Check sheet for the drawn part. Datum: minimum x, y, z corner. Units: mm. Round coordinates to 2 decimals unless told otherwise and drop trailing zeros. Write each loop counter-clockwise with the first axis right and the second up, starting at its lowest first coordinate (ties: lowest second). Pieces come first, ordered by that corner, then holes. Notation, with made-up numbers: (79, 18) -> (138, 18) arc R13 cw to (138, 28) -> close; hole circle Ø10 at (-3.5, 0.5). An arc over 180 degrees is marked (long way). One line per item, written item: value.
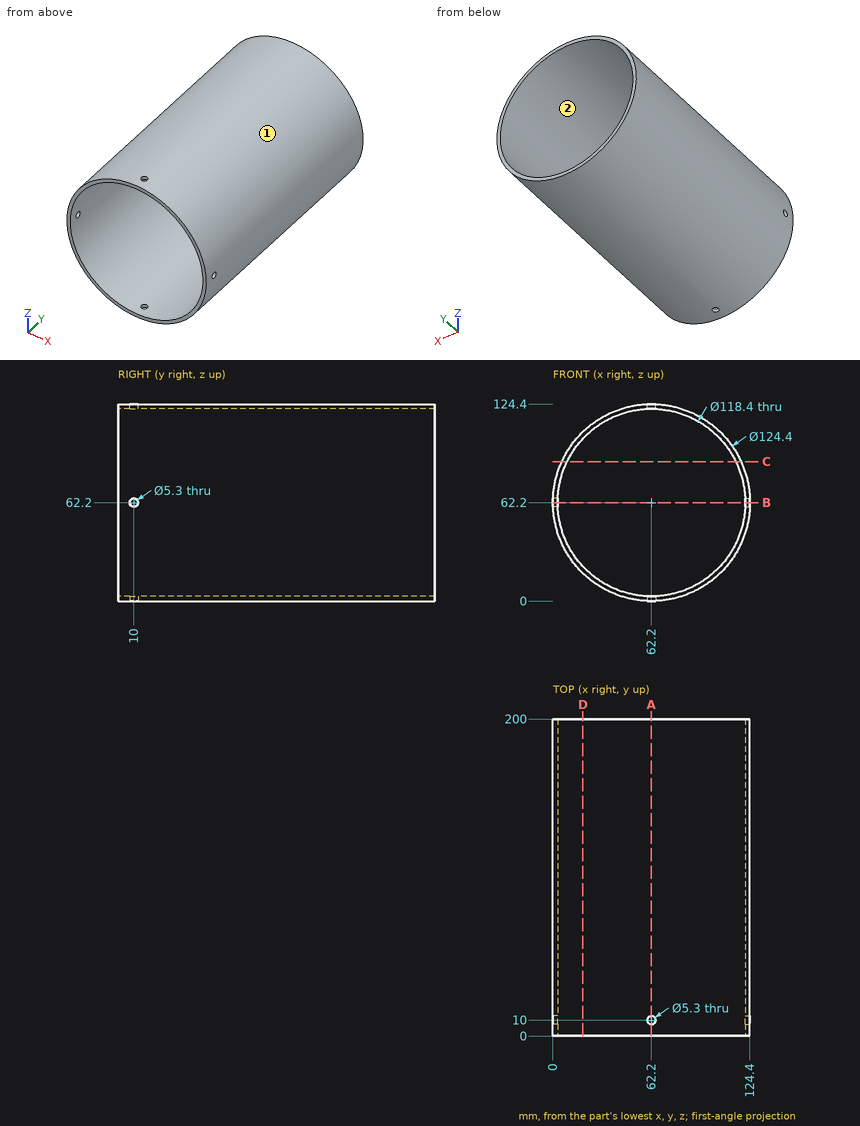
Item 1: Thickness scan on line 1 (X direction, y = 69.5, z = 62.2); line 2 (Y direction, x = 0.85, z = 62.2); line 3 (Z direction, x = 116, y = 17). Record the ranges inside material, lowest first.
Answer:
line 1: x = 0 to 3, 121.4 to 124.4
line 2: y = 0 to 7.35, 12.65 to 200
line 3: z = 30.98 to 37.5, 86.9 to 93.42
Item 2: Sectioned sample at B-B on z = 62.2. Enter the section's corners in (x, y).
Answer:
outline: (0, 0) -> (3, 0) -> (3, 7.35) -> (0, 7.35) -> close; (0, 12.65) -> (3, 12.65) -> (3, 200) -> (0, 200) -> close; (121.4, 0) -> (124.4, 0) -> (124.4, 7.35) -> (121.4, 7.35) -> close; (121.4, 12.65) -> (124.4, 12.65) -> (124.4, 200) -> (121.4, 200) -> close
Item 3: Mould release check, pull along X, two halves, no side actions. Record for the marked faces 1 and 2: pulls with the +X half, pulls with the -X half, needs draft (parallel to the pull), parting line crosses it, or undercut.
Answer:
face 1: parting line crosses it
face 2: undercut
Item 4: Sectioned sample at A-A on x = 62.2. Enter the section's corners in (y, z).
Answer:
outline: (0, 0) -> (7.35, 0) -> (7.35, 3) -> (0, 3) -> close; (0, 121.4) -> (7.35, 121.4) -> (7.35, 124.4) -> (0, 124.4) -> close; (12.65, 0) -> (200, 0) -> (200, 3) -> (12.65, 3) -> close; (12.65, 121.4) -> (200, 121.4) -> (200, 124.4) -> (12.65, 124.4) -> close
Item 5: Sectioned sample at D-D on x = 19. Enter the section's corners in (y, z).
Answer:
outline: (0, 17.45) -> (200, 17.45) -> (200, 21.72) -> (0, 21.72) -> close; (0, 102.68) -> (200, 102.68) -> (200, 106.95) -> (0, 106.95) -> close
Item 6: Sectioned sample at C-C on z = 88. Enter the section's corners in (x, y).
Answer:
outline: (5.6, 0) -> (8.92, 0) -> (8.92, 200) -> (5.6, 200) -> close; (115.48, 0) -> (118.8, 0) -> (118.8, 200) -> (115.48, 200) -> close
Item 7: Depth check by flat-ended pin: P1, Ø12, axis at x = 44, y = 122.5, coming from the -Z side; P2, Ø10, axis at x = 72.5, y = 139, coming from the -Z side; P3, Ø3, axis at x = 52, y = 92.5, coming from the -Z side. Enter the tip coordinate at first touch or a pass-through.
Answer:
P1: stops at z = 1.21
P2: stops at z = 0.23
P3: stops at z = 0.61
